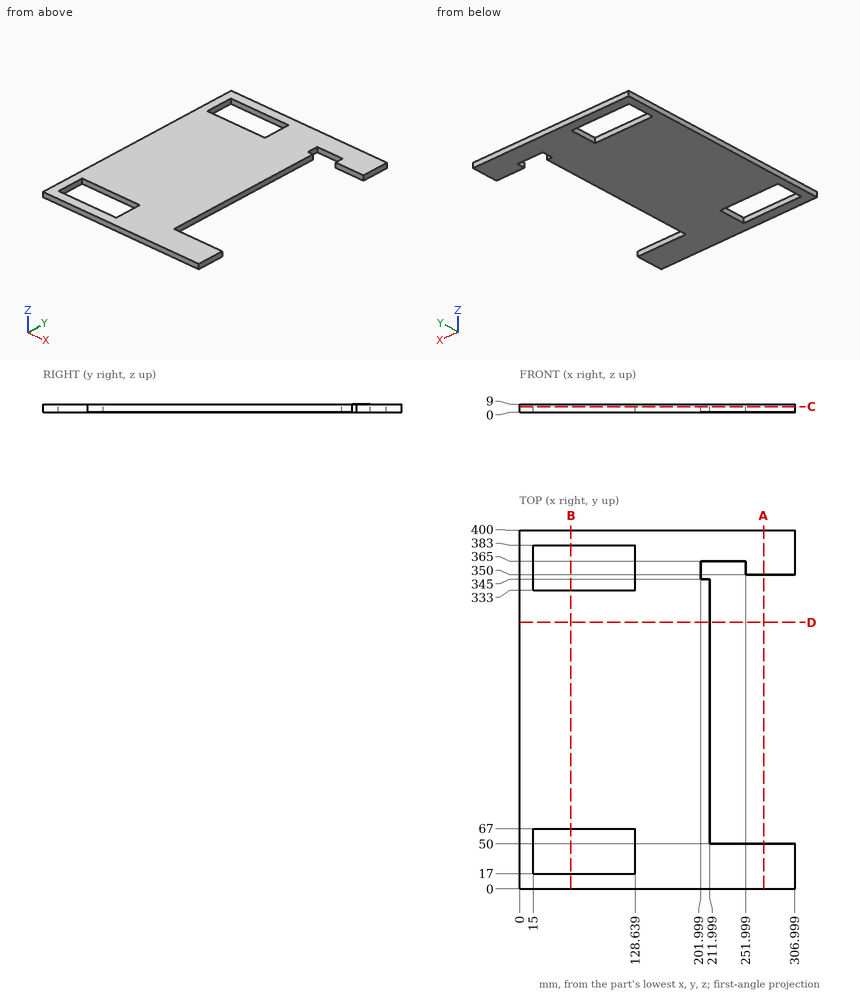
Print and shaded views of the part. All mm, measured from the part's lowest x, y and z. Give positions to 0.01 mm unless a question says otherwise; leave off trailing zeros. Write each loop counter-clockwise with the first axis right and the second up, starting at its lowest first coordinate (ties: lowest second). Pieces come first, ordered by that corner, then holes. Notation, with made-up numbers: (4.25, -23) -> (48.25, -23) arc R12 cw to (48.25, -1) -> close; hole circle Ø10 at (42.25, 38.5). An arc over 180 degrees is marked (long way). Use CSV: the item, a comma, the result in double quotes. Start each with the question number.
1) Cut at D-D on y = 297. List the corners of the cut face in (x, z), plus the area to 3 significant figures.
2) Cut at C-C on z = 6. List the corners of the cut face in (x, y).
3) Cut at A-A on x = 272. List the corners of the cut face in (y, z), plus the area to 3 significant figures.
4) Drill centre lines: L1, parallel to Y at x = 65, z = 6.5; L2, parallel to X at y = 37, z = 5; L3, parallel to Y at x = 266, z = 8.5. Where is each one in solid material? Low to high.
5) Cut at B-B on x = 57. List the corners of the cut face in (y, z), plus the area to 3 significant figures.
6) Pin check, flat tip, straight feed: P1, Ø2.5, axis at y = 129.5, z = 2.5, coming from the +X side. Stop position of the tip, or through.
Final values:
1,outline,"(0, 0) -> (212, 0) -> (212, 9) -> (0, 9) -> close"
1,area,"1,910 mm2"
2,outline,"(0, 0) -> (307, 0) -> (307, 50) -> (212, 50) -> (212, 345) -> (202, 345) -> (202, 365) -> (252, 365) -> (252, 350) -> (307, 350) -> (307, 400) -> (0, 400) -> close; hole (15, 17) -> (128.64, 17) -> (128.64, 67) -> (15, 67) -> close; hole (15, 333) -> (128.64, 333) -> (128.64, 383) -> (15, 383) -> close"
3,outline,"(0, 0) -> (50, 0) -> (50, 9) -> (0, 9) -> close; (350, 0) -> (400, 0) -> (400, 9) -> (350, 9) -> close"
3,area,"900 mm2"
4,L1,"y = 0 to 17, 67 to 333, 383 to 400"
4,L2,"x = 0 to 15, 128.64 to 307"
4,L3,"y = 0 to 50, 350 to 400"
5,outline,"(0, 0) -> (17, 0) -> (17, 9) -> (0, 9) -> close; (67, 0) -> (333, 0) -> (333, 9) -> (67, 9) -> close; (383, 0) -> (400, 0) -> (400, 9) -> (383, 9) -> close"
5,area,"2,700 mm2"
6,P1,"stops at x = 212"
